```python
from build123d import *

# Parameters (mm, degrees)
SKETCH_1_W         = 20
SKETCH_1_H         = 20
SKETCH_1_W_2       = 16
SKETCH_1_H_2       = 16
EXTRUDE_1_DEPTH    = 550
SKETCH1_R          = 2
CUT_EXTRUDE1_DEPTH = 20
SKETCH2_R          = 2.5
CUT_EXTRUDE2_DEPTH = 20
SKETCH5_R          = 1.5
CUT_EXTRUDE3_DEPTH = 20


with BuildPart() as part:
    # 草图1 → 凸台-拉伸1 (new body)
    with BuildSketch(Plane.XY):
        Rectangle(SKETCH_1_W, SKETCH_1_H)
        Rectangle(SKETCH_1_W_2, SKETCH_1_H_2, mode=Mode.SUBTRACT)
    extrude(amount=EXTRUDE_1_DEPTH)

    # Sketch1 → Cut-Extrude1 (cut)
    with BuildSketch(Plane.ZY.offset(10)):
        with Locations((532.5, 0)):
            Circle(SKETCH1_R)
        with Locations((517.5, 0)):
            Circle(SKETCH1_R)
    extrude(amount=-CUT_EXTRUDE1_DEPTH, mode=Mode.SUBTRACT)

    # Sketch2 → Cut-Extrude2 (cut)
    with BuildSketch(Plane.ZY.offset(10)):
        with Locations((10, 0)):
            Circle(SKETCH2_R)
        with Locations((30, 0)):
            Circle(SKETCH2_R)
        with Locations((50, 0)):
            Circle(SKETCH2_R)
    extrude(amount=-CUT_EXTRUDE2_DEPTH, mode=Mode.SUBTRACT)

    # Sketch5 → Cut-Extrude3 (cut)
    with BuildSketch(Plane.XZ.offset(10)):
        with Locations(Location((0, 482.5, 0), (0, 0, 270))):
            Circle(SKETCH5_R)
        with Locations(Location((0, 462.5, 0), (0, 0, 270))):
            Circle(SKETCH5_R)
        with Locations(Location((0, 362.5, 0), (0, 0, 270))):
            Circle(SKETCH5_R)
        with Locations(Location((0, 342.5, 0), (0, 0, 270))):
            Circle(SKETCH5_R)
        with Locations(Location((0, 242.5, 0), (0, 0, 270))):
            Circle(SKETCH5_R)
        with Locations(Location((0, 222.5, 0), (0, 0, 270))):
            Circle(SKETCH5_R)
        with Locations(Location((0, 122.5, 0), (0, 0, 270))):
            Circle(SKETCH5_R)
        with Locations(Location((0, 102.5, 0), (0, 0, 270))):
            Circle(SKETCH5_R)
    extrude(amount=-CUT_EXTRUDE3_DEPTH, mode=Mode.SUBTRACT)


solid = part.part
```
The model under review builds one solid part; all positions refer to its coordinate system, in mm. A direction names the side the tool comes from. Round coordinates to 2 decimals unless told otherwise and drop trailing zeros. Order: outer loops, then holes, each group sorted by start corner. A loop starts at its lowest first (then second) coordinate and runs counter-clockwise, first axis right, second up. Notation, with made-up numbers: (36, 81.5) - (66, 81.5) arc R30 ccw to (66, 106.5) - close; hole circle Ø10 at (4.25, -9). An arc over 180 degrees is marked (long way). Answer in a Markdown table with one row per item.
(1) Take a section at A-A on z = 92. Write out the cut boundary in (x, y), plus the area to 3 significant figures.
Result set:
| item | result |
|---|---|
| outline | (-10, -10) - (10, -10) - (10, 10) - (-10, 10) - close; hole (-8, -8) - (8, -8) - (8, 8) - (-8, 8) - close |
| area | 144 mm2 |
(2) Machinability: for faces 1 (the face through (-8, 0, 271)), 2 (the face through (-10, 0, 271)), which of the approach directions +Z, -Z, +X, -X, +Y, -Y give a long, thin tool a straight path to every point of the face, cutting with its end or side? Answer none if there is none.
Result set:
| item | result |
|---|---|
| face 1 | +Z, -Z |
| face 2 | +Z, -Z, -X, +Y, -Y |
(3) Clearance check with a flat-ended pin moving along its axis: P1, Ø10, axis at x = -1, y = 2.5, coming from the -Z side. State where the tip first meets the part, or that it passes through.
Result set:
| item | result |
|---|---|
| P1 | passes through |
(4) Take a section at B-B on x = 4.5. Write out the cut boundary in (y, z), plus the area to 3 significant figures.
Result set:
| item | result |
|---|---|
| outline | (-10, 0) - (-8, 0) - (-8, 550) - (-10, 550) - close; (8, 0) - (10, 0) - (10, 550) - (8, 550) - close |
| area | 2,200 mm2 |
(5) Mouldability with a two-part tool opening along Y and no side actions: class faces 3 (the face through (0, -8, 271)), 4 (the face through (0, 8, 271)), 5 (the face through (-9, 0, 0)), 6 (the face through (0, -10, 271)) as released by +Y, released by -Y, zero draft, split by the parting line, or undercut.
Result set:
| item | result |
|---|---|
| face 3 | undercut |
| face 4 | undercut |
| face 5 | zero draft |
| face 6 | released by -Y |
(6) For line 1 (X direction, y = 4.25, z = 189); line 2 (X direction, y = -8.75, z = 102.5), list the stretches that pass through material, from the lowest coordinate up. Write a range as from..to.
Result set:
| item | result |
|---|---|
| line 1 | x = -10..-8, 8..10 |
| line 2 | x = -10..-1.5, 1.5..10 |
